```python
from build123d import *

# Parameters (mm, degrees)
F1_DEPTH = 25.4
F2_D     = 5.1054
F2_DEPTH = 15.875
F2_TIP   = 1.5338169022
F3_W     = 6.35
F3_H     = 7.2735160964
F4_DEPTH = 2.2235
F6_D     = 3.4544


with BuildPart() as f1:
    # F0 (on Front) → F1 (new body)
    with BuildSketch(Plane.XZ):
        with BuildLine():
            ThreePointArc((1.5875, -3.4635160964), (3.2065928179, -2.0576351717), (3.81, 0))
            ThreePointArc((3.81, 0), (-2.0576351717, 3.2065928179), (-1.5875, -3.4635160964))
            Line((-1.5875, -3.4635160964), (-1.5875, 0))
            Line((-1.5875, 0), (1.5875, 0))
            Line((1.5875, 0), (1.5875, -3.4635160964))
        make_face()
        with BuildLine():
            Line((-1.5875, 0), (-1.5875, -3.4635160964))
            ThreePointArc((-1.5875, -3.4635160964), (0, -3.81), (1.5875, -3.4635160964))
            Line((1.5875, -3.4635160964), (1.5875, 0))
            Line((1.5875, 0), (-1.5875, 0))
        make_face()
        with BuildLine():
            ThreePointArc((1.5875, -3.4635160964), (0, -3.81), (-1.5875, -3.4635160964))
            Line((-1.5875, -3.4635160964), (-1.5875, -9.525))
            Line((-1.5875, -9.525), (1.5875, -9.525))
            Line((1.5875, -9.525), (1.5875, -3.4635160964))
        make_face()
    extrude(amount=-F1_DEPTH)

    # F2
    with Locations(Plane.XZ):
        with Locations((0, 0)):
            Hole(F2_D / 2, depth=F2_DEPTH)
            with Locations((0, 0, -(F2_DEPTH + F2_TIP / 2))):  # 118° drill point
                Cone(0, F2_D / 2, F2_TIP, mode=Mode.SUBTRACT)

    # F3 (on face) → F4 (cut, through all)
    with BuildSketch(Plane.YZ.offset(1.5875)):
        with Locations((22.225, 0.1732419518)):
            Rectangle(F3_W, F3_H)
    extrude(amount=F4_DEPTH, mode=Mode.SUBTRACT)

    # F6 (through all)
    with Locations(Plane.YZ.offset(1.5875)):
        with Locations((22.225, 0.1442580482), (22.225, -6.2057419518)):
            Hole(F6_D / 2)


solid = f1.part
```
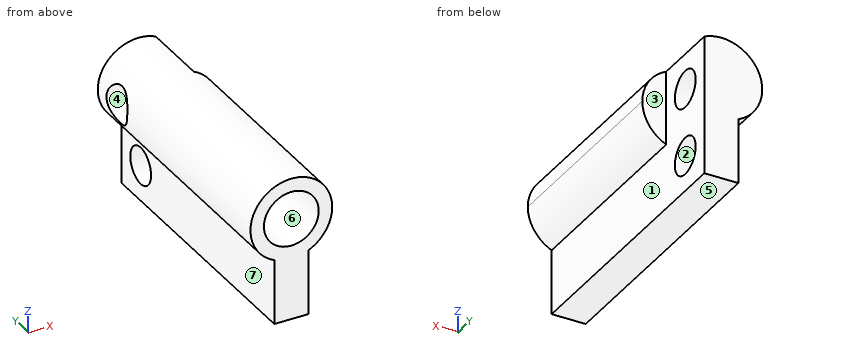
Check sheet for the modelled part. Datum: model origin and axes. Units: mm. Face numbers are marked on the shaded views. A direction names the side the tool comes from. Coordinates: 2 decimals unless noted, no trailing zeros. Order: outer loops, then holes, each group sorted by start corner. A loop starts at its lowest first (then second) coordinate and runs counter-clockwise, first axis right, second up. Notation, with made-up numbers: (21.25, 60.25) -> (60.25, 60.25) arc R15 cw to (60.25, 88.25) -> close; hole circle Ø10 at (-22.75, 83). An arc over 180 degrees is marked (long way). Write each question's results on one line, items separated by ' | '. Start each with the question number.
1) Section check A-A (y = 3). Enter the section's corners in (x, z) (1 decimal), and give its area (3 significant figures).
2) Draft check along Z on the marked faces 4, 5, 6 and 7. Enter one of: pulls with the +Z half, pulls with the -Z half, needs draft (parallel to the pull), parting line crosses it, or undercut.
3) Section check C-C (x = -3). Enter the section's corners in (y, z) (3 decimals).
4) Material ranges on line 1 along Z through (x, y) = (0, 11.5) (3 decimals); line 2 along X through (y, z) = (19.25, -6); line 3 along Z through (x, y) = (-2.75, 22.25), recorded low to high.
5) Set-up check for the marked faces 1, 2 and 3: record each of +Z, -Z, +X, -X, +Y, -Y from which the full face is reachable in a straight line by a thin tool's end or side.
6) Section check B-B (y = 21). Enter the section's corners in (x, z) (1 decimal).
7) Section check D-D (z = -3.75). Enter the section's corners in (x, y), and give its area (3 significant figures).
8) Depth check by flat-ended pin: pin 1 (3 mm diameter, centred on y = 5, z = 2.5, fed in from +X); pin 2 (1 mm diameter, centred on y = 7, z = -2.5, fed in from -X); pin 3 (6.5 mm diameter, centred on y = 17, z = -7, fed in from -X). Enter the tip coordinate at first touch or a pass-through.
Checked values:
1) outline: (-1.6, -9.5) -> (1.6, -9.5) -> (1.6, -3.5) arc R3.8 ccw (long way) to (-1.6, -3.5) -> close; hole circle Ø5.1 at (0, 0) | area: 43.6 mm²
2) face 4: undercut | face 5: pulls with the -Z half | face 6: undercut | face 7: needs draft
3) outline: (0, -2.349) -> (25.4, -2.349) -> (25.4, 2.349) -> (0, 2.349) -> close; hole circle Ø3.454 at (22.225, 0.144)
4) line 1: -9.525 to -2.553, 2.553 to 3.81 | line 2: -1.59 to 1.59 | line 3: -2.64 to -1.58, 1.87 to 2.64
5) face 1: -Z, +X, +Y | face 2: +X, -X | face 3: +Z, -Z, +X, +Y
6) outline: (-3.7, -1.1) arc R3.8 ccw to (-1.6, -3.5) -> (-1.6, -5) -> (1.6, -5) -> (1.6, -1.1) -> close; (-3.6, 1.4) -> (1.6, 1.4) -> (1.6, 3.5) arc R3.8 ccw to start; (-1.6, -9.5) -> (1.6, -9.5) -> (1.6, -7.4) -> (-1.6, -7.4) -> close
7) outline: (-1.59, 0) -> (1.59, 0) -> (1.59, 25.4) -> (-1.59, 25.4) -> close | area: 80.6 mm²
8) pin 1: x = 3.68 | pin 2: x = -3.24 | pin 3: x = -1.59
